Autodesk Inventor part; units mm, degrees
ref_plane "YZ Plane" through (0, 0, 0) normal (1, 0, 0) x (0, 1, 0)
ref_plane "XZ Plane" through (0, 0, 0) normal (0, 1, 0) x (-1, 0, 0)
ref_plane "XY Plane" through (0, 0, 0) normal (0, 0, 1) x (1, 0, 0)
sketch "Sketch1" plane through (0, 0, 0) normal (0, 0, 1) x (1, 0, 0)
  circle A0 centre (0, 0) radius 1.5
  circle A1 centre (0, 0) radius 4
  dimension "d0" = 3
  dimension "d1" = 8
extrude "Extrusion1" add sketch "Sketch1" along normal blind 4
sketch "Sketch2" plane through (0, 0, 4) normal (0, 0, 1) x (1, 0, 0)
  circle A0 centre (0, 0) radius 1.5
  circle A1 centre (0, 0) radius 4
  circle A2 centre (0, 0) radius 2.25
  circle A3 centre (0, 0) radius 3.25
  dimension "d4" = 0.75
  dimension "d5" = 0.75
extrude "Extrusion2" cut sketch "Sketch2" against normal blind 0.25 contours A3
sketch "Sketch3" plane through (0, 0, 0) normal (0, 0, -1) x (-1, 0, 0)
  circle A0 centre (0, 0) radius 1.5
  circle A1 centre (0, 0) radius 4
  circle A2 centre (0, 0) radius 2.25
  circle A3 centre (0, 0) radius 3.25
  dimension "d8" = 0.75
  dimension "d9" = 0.75
extrude "Extrusion3" cut sketch "Sketch3" against normal blind 0.25 contours A3
chamfer "Chamfer1" distance 0.1 angle 45 2 edges at (-4, 0, 4) (-4, 0, 0)
properties part number "3x8x4_bearing"
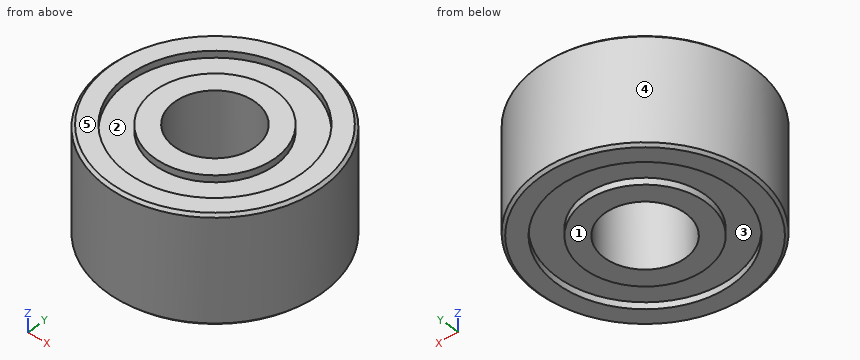
Work out the finished part from the listing and answer in its coordinate system (mm). Face numbers are marked on the shaded views. A direction names the side the tool comes from. Round coordinates to 2 decimals unless told otherwise and drop trailing zeros. Loops run counter-clockwise (first coordinate to the right, second up) from the corner with the lowest first, then second, coordinate; pieces in that order, holes last.
(1) Each of these flat-tipped pins is pushed along its axis until it touches: P1, Ø1, axis at y = 3, z = 2.5, coming from the +X side; P2, Ø4, axis at x = 0, y = 0, coming from the +Z side. Where does it stop, or does it pass through?
Computed values:
P1: stops at x = 3.12
P2: stops at z = 4
(2) For the marked faces 1 and 2, determine the directions among +Z, -Z, +X, -X, +Y, -Y from which every point of the face is accessible in a straight line to the end or side of a thin tool.
Computed values:
face 1: -Z, +X, -X, +Y, -Y
face 2: +Z
(3) The part is cut by section A-A, the plane x = 0. Give the vertices of the cut face in (y, z), and give its area (3 significant figures).
Computed values:
outline: (-4, 0.1) - (-3.9, 0) - (-3.25, 0) - (-3.25, 0.25) - (-2.25, 0.25) - (-2.25, 0) - (-1.5, 0) - (-1.5, 4) - (-2.25, 4) - (-2.25, 3.75) - (-3.25, 3.75) - (-3.25, 4) - (-3.9, 4) - (-4, 3.9) - close; (1.5, 0) - (2.25, 0) - (2.25, 0.25) - (3.25, 0.25) - (3.25, 0) - (3.9, 0) - (4, 0.1) - (4, 3.9) - (3.9, 4) - (3.25, 4) - (3.25, 3.75) - (2.25, 3.75) - (2.25, 4) - (1.5, 4) - close
area: 19.0 mm2
(4) The mould has two halves that part along X. Classify the marked faces 3, 4 and 5: pulls with the +X half, pulls with the -X half, needs draft (parallel to the pull), parting line crosses it, or undercut.
Computed values:
face 3: undercut
face 4: parting line crosses it
face 5: needs draft
(5) Find the intervals of material crossed by L1, parallel to Y at x = 0, z = 3.85; L2, parallel to Y at x = 0, z = 1.25; L3, parallel to Y at x = 0, z = 3.95, in increasing order.
Computed values:
L1: y = -4 to -3.25, -2.25 to -1.5, 1.5 to 2.25, 3.25 to 4
L2: y = -4 to -1.5, 1.5 to 4
L3: y = -3.95 to -3.25, -2.25 to -1.5, 1.5 to 2.25, 3.25 to 3.95
(6) The part is cut by section C-C, the plane z = 1.8. Give the vertices of the cut face in (x, y).
Computed values:
outline: circle Ø8 at (0, 0); hole circle Ø3 at (0, 0)
